Check sheet for the modelled part. Datum: model origin and axes. Units: mm. A direction names the side the tool comes from. Round coordinates to 2 decimals unless told otherwise and drop trailing zeros. Write each loop counter-clockwise with the first axis right and the second up, starting at its lowest first coordinate (ties: lowest second). Pieces come first, ordered by that corner, then holes.
Item 1: Release check for a two-part mould opening along Y. For faces 5 (the flat face through (0, -8, 0)), 6 (the flat face through (5.3, -3, -7.5)), 7 (the flat face through (0, -5, 8)), 8 (the flat face through (0, -1.6, -7.5)) record: +Y half, -Y half, draft (parallel to the pull), parting line (faces both ways), or undercut.
Item 2: Material ranges on line 1 (X direction, y = -3.25, z = -7); line 2 (Z direction, x = 6.25, y = -0.25), recorded low to high.
Item 3: Cross-section at B-B on z = 0.5. Enter the section's corners in (x, y).
Item 4: Tool access check on faces 1 (the flat face through (-4.7, -3, 7.5)), 2 (the flat face through (7, -1, 0)), 3 (the cylindrical face through (7.469, -5.465, -7.686)), 4 (the flat face through (0, -1.6, 7.5)). Record the directions out of +Z, -Z, +X, -X, +Y, -Y that give a thin tool (end or side, any length) a straight path to the whole face; none if there is none.
Item 5: Go/stop test with flat-tipped pins: pin 1 Ø1.5 at (y, z) = (-2, -0.5) entering from +X; pin 2 Ø1.1 at (x, y) = (4, 0.5) entering from +Z; pin 3 Ø0.5 at (x, y) = (-2, 0.5) entering from -Z. Record where each tip stops, or that it passes through.
Item 6: Cross-section at D-D on y = -1. Enter the section's corners in (x, z) (3 decimals).
Item 7: Cross-section at C-C on x = -2.75. Enter the section's corners in (y, z).
from build123d import *

# Parameters (mm, degrees)
SKETCH2_W           = 15.6
SKETCH2_H           = 15.6
BOSS_EXTRUDE2_DEPTH = 1
BOSS_EXTRUDE1_DEPTH = 3
SKETCH3_W           = 4.6
SKETCH3_H           = 1
BOSS_EXTRUDE3_DEPTH = 1.4
FILLET1_R           = 0.755
BOSS_EXTRUDE4_DEPTH = 5


with BuildPart() as part:
    # Sketch2 → Boss-Extrude2 (new body)
    with BuildSketch(Plane(origin=(0, 0, 0), x_dir=(1, 0, 0), z_dir=(0, 1, 0))):
        Rectangle(SKETCH2_W, SKETCH2_H)
    extrude(amount=BOSS_EXTRUDE2_DEPTH)

    # Cutout → Boss-Extrude1 (add)
    with BuildSketch(Plane(origin=(0, 0, 0), x_dir=(1, 0, 0), z_dir=(0, 1, 0))):
        Polygon((-7.8, 3), (-7, 3), (-7, -3), (-7.8, -3), (-7.8, -7), (7.8, -7), (7.8, -3), (7, -3), (7, 3), (7.8, 3), (7.8, 7), (-7.8, 7), align=None)
    extrude(amount=-BOSS_EXTRUDE1_DEPTH)

    # Sketch3 → Boss-Extrude3 (add)
    with BuildSketch(Plane(origin=(0, -1.6, 0), x_dir=(-1, 0, 0), z_dir=(0, 1, 0))):
        with Locations((0, 7.5)):
            Rectangle(SKETCH3_W, SKETCH3_H)
    boss_extrude3 = extrude(amount=-BOSS_EXTRUDE3_DEPTH)

    # Mirror1: Boss-Extrude3 across plane
    add(boss_extrude3.mirror(Plane.XY))

    # Fillet1
    fillet1_edges = [part.edges().sort_by_distance(p)[0] for p in [
        (7.8, -1.5, 7),
        (7.8, -1.5, 3),
        (7.8, -1.5, -3),
        (7.8, -1.5, -7),
        (2.3, -2.3, -8),
        (-2.3, -2.3, -8),
        (-7.8, -1.5, -3),
        (-7.8, -1.5, -7),
        (2.3, -2.3, 8),
        (-2.3, -2.3, 8),
        (-7.8, -1.5, 7),
        (-7.8, -1.5, 3),
    ]]
    fillet(fillet1_edges, radius=FILLET1_R)

    # Sketch4 → Boss-Extrude4 (add)
    with BuildSketch(Plane.XZ.offset(3)):
        with BuildLine():
            Line((-6.7, -8), (6.7, -8))
            ThreePointArc((6.7, -8), (7.477817459, -7.677817459), (7.8, -6.9))
            Line((7.8, -6.9), (7.8, 6.9))
            ThreePointArc((7.8, 6.9), (7.477817459, 7.677817459), (6.7, 8))
            Line((6.7, 8), (-6.7, 8))
            ThreePointArc((-6.7, 8), (-7.477817459, 7.677817459), (-7.8, 6.9))
            Line((-7.8, 6.9), (-7.8, -6.9))
            ThreePointArc((-7.8, -6.9), (-7.477817459, -7.677817459), (-6.7, -8))
        make_face()
    extrude(amount=BOSS_EXTRUDE4_DEPTH)


solid = part.part
Response values:
1. face 5: -Y half
1. face 6: undercut
1. face 7: draft
1. face 8: undercut
2. line 1: x = -7.8 to 7.8
2. line 2: z = -7 to 7
3. outline: (-7.8, -8) - (7.8, -8) - (7.8, -3) - (7, -3) - (7, 0) - (7.8, 0) - (7.8, 1) - (-7.8, 1) - (-7.8, 0) - (-7, 0) - (-7, -3) - (-7.8, -3) - close
4. face 1: +Z, -X
4. face 2: +X
4. face 3: -Z, +X, -Y
4. face 4: +Z, +X, -X
5. pin 1: stops at x = 7
5. pin 2: stops at z = 7.8
5. pin 3: stops at z = -7.8
6. outline: (-7.8, -6.245) arc R0.755 ccw to (-7.045, -7) - (7.045, -7) arc R0.755 ccw to (7.8, -6.245) - (7.8, -3.755) arc R0.755 ccw to (7.045, -3) - (7, -3) - (7, 3) - (7.045, 3) arc R0.755 ccw to (7.8, 3.755) - (7.8, 6.245) arc R0.755 ccw to (7.045, 7) - (-7.045, 7) arc R0.755 ccw to (-7.8, 6.245) - (-7.8, 3.755) arc R0.755 ccw to (-7.045, 3) - (-7, 3) - (-7, -3) - (-7.045, -3) arc R0.755 ccw to (-7.8, -3.755) - close
7. outline: (-8, -8) - (-3, -8) - (-3, -7) - (0, -7) - (0, -7.8) - (1, -7.8) - (1, 7.8) - (0, 7.8) - (0, 7) - (-3, 7) - (-3, 8) - (-8, 8) - close
